Job drawing, mm, ordinate dimensions from the low corner. One solid piece. Give positions to 0.01 mm unless a question says otherwise; leave off trailing zeros. Write each loop counter-clockwise with the first axis right and the second up, starting at its lowest first coordinate (ties: lowest second). Pieces come first, ordered by that corner, then holes. Notation, with made-up numbers: (73.5, -13) - (113.5, -13) arc R21 ccw to (113.5, 5) - close; hole circle Ø3 at (-5, 62.25). An arc over 180 degrees is marked (long way). Answer in a Markdown table with one row per item. Add a question column.
1. Probe line 1 along X through (y, z) = (21.5, 1.25); line 2 along Y through (x, z) = (21, 6); line 3 along Z through (x, y) = (35, 21.5). List the from-to ranges inside material, lowest first.
2. Band-saw the part on B-B on x = 22. Write the cut outline in (y, z).
3. Pull direction Y, two halves, no side cores. Call the marked faces 1, 2, 3 and 4: released by +Y, released by -Y, zero draft, split by the parting line, or undercut.
4. Band-saw the part on A-A on z = 1.25. Write the cut outline in (x, y), plus the area to 3 significant figures.
5. Band-saw the part on D-D on x = 13. Write the cut outline in (y, z), plus the area to 3 significant figures.
6. Band-saw the part on C-C on y = 22. Write the cut outline in (x, z), plus the area to 3 significant figures.
7. Drop flat-ended pins along their axis: pin 1 Ø1.8 at (x, y) = (22, 22) entering from +Z; pin 2 Ø2 at (x, z) = (5.5, 6.5) entering from +Y; pin 3 Ø1.5 at (x, z) = (28.5, 5.5) entering from -Y; pin 4 Ø3 at (x, z) = (17.5, 6) entering from +Y. Give the stop position or say it passes through.
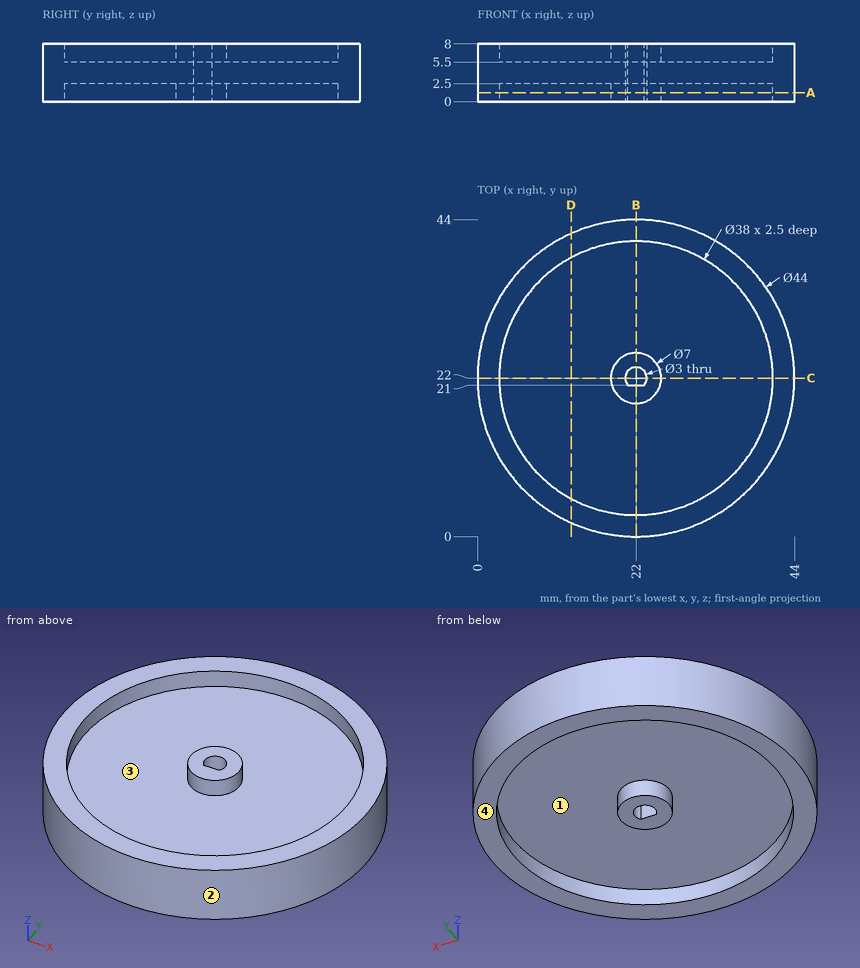
Values:
| question | item | result |
|---|---|---|
| 1 | line 1 | x = 0.01 to 3.01, 18.54 to 20.59, 23.41 to 25.46, 40.99 to 43.99 |
| 1 | line 2 | y = 0.02 to 3.03, 18.65 to 21, 23.12 to 25.35, 40.97 to 43.98 |
| 1 | line 3 | z = 2.5 to 5.5 |
| 2 | outline | (0, 0) - (3, 0) - (3, 2.5) - (18.5, 2.5) - (18.5, 0) - (21, 0) - (21, 8) - (18.5, 8) - (18.5, 5.5) - (3, 5.5) - (3, 8) - (0, 8) - close; (23.5, 0) - (25.5, 0) - (25.5, 2.5) - (41, 2.5) - (41, 0) - (44, 0) - (44, 8) - (41, 8) - (41, 5.5) - (25.5, 5.5) - (25.5, 8) - (23.5, 8) - close |
| 3 | face 1 | undercut |
| 3 | face 2 | split by the parting line |
| 3 | face 3 | undercut |
| 3 | face 4 | zero draft |
| 4 | outline | circle Ø44 at (22, 22); circle Ø7 at (22, 22); hole circle Ø38 at (22, 22); hole (20.88, 21) - (23.12, 21) arc R1.5 ccw (long way) to start |
| 4 | area | 419 mm² |
| 5 | outline | (1.93, 0) - (5.27, 0) - (5.27, 2.5) - (38.73, 2.5) - (38.73, 0) - (42.07, 0) - (42.07, 8) - (38.73, 8) - (38.73, 5.5) - (5.27, 5.5) - (5.27, 8) - (1.93, 8) - close |
| 5 | area | 154 mm² |
| 6 | outline | (0, 0) - (3, 0) - (3, 2.5) - (18.5, 2.5) - (18.5, 0) - (20.5, 0) - (20.5, 8) - (18.5, 8) - (18.5, 5.5) - (3, 5.5) - (3, 8) - (0, 8) - close; (23.5, 0) - (25.5, 0) - (25.5, 2.5) - (41, 2.5) - (41, 0) - (44, 0) - (44, 8) - (41, 8) - (41, 5.5) - (25.5, 5.5) - (25.5, 8) - (23.5, 8) - close |
| 6 | area | 173 mm² |
| 7 | pin 1 | passes through |
| 7 | pin 2 | stops at y = 37.61 |
| 7 | pin 3 | stops at y = 0.76 |
| 7 | pin 4 | stops at y = 43.79 |
